Autodesk Inventor part; units mm, degrees
ref_plane "YZ Plane" through (0, 0, 0) normal (1, 0, 0) x (0, 1, 0)
ref_plane "XZ Plane" through (0, 0, 0) normal (0, 1, 0) x (-1, 0, 0)
ref_plane "XY Plane" through (0, 0, 0) normal (0, 0, 1) x (1, 0, 0)
sketch "Sketch1" plane through (0, 0, 0) normal (0, 1, 0) x (-1, 0, 0)
  line L0 (14.85, 7) -> (10.15, 7)
  line L1 (10.15, 7) -> (10.15, 2)
  line L2 (10.15, 2) -> (-10.15, 2)
  line L3 (-10.15, 2) -> (-10.15, 7)
  line L4 (-10.15, 7) -> (-14.85, 7)
  line L5 (-14.85, 7) -> (-14.85, 5)
  line L6 (-14.85, 5) -> (-12.15, 5)
  line L7 (-12.15, 5) -> (-12.15, 0)
  line L8 (-12.15, 0) -> (12.15, 0)
  line L9 (12.15, 0) -> (12.15, 5)
  line L10 (12.15, 5) -> (14.85, 5)
  line L11 (14.85, 5) -> (14.85, 7)
  point P0 (0, 0)
  point P1 (0, 0)
  point P2 (0, 2)
  point P3 (12.5, 7)
  point P4 (13.5, 5)
  dimension "d0" = 20.3
  dimension "d1" = 24.3
  dimension "d2" = 5
  dimension "d3" = 4.7
  dimension "d5" = 2
  dimension "d6" = 2
extrude "Extrusion1" add sketch "Sketch1" along normal mid plane 50
sketch "Sketch2" plane through (-10.15, 25, 2) normal (0, 0, 1) x (1, 0, 0)
  line L0 (13.1499, -10.0316) -> (13.1499, -19.0316)
  line L1 (7.1499, -19) -> (7.1499, -10)
  arc A0 (13.1499, -10.0316) -> (7.1499, -10) centre (10.15, -10) ccw
  arc A1 (7.1499, -19) -> (13.1499, -19.0316) centre (10.15, -19) ccw
  line L2 (0, 0) -> (20.3, 0)
  point P0 (10.15, -25)
  dimension "d9" = 6
  dimension "d12" = 9
  dimension "d13" = 10
extrude "Extrusion2" cut sketch "Sketch2" against normal up to surface (2 mm away)
pattern_linear "Rectangular Pattern1" count 2 spacing 25 along (0, -1, 0) of "Extrusion2"
properties part number "Part_B8"
Geometry check sheet. Reference: the model listing, model coordinates, mm. A direction names the side the tool comes from. Coordinates: 2 decimals unless noted, no trailing zeros. Write each loop counter-clockwise with the first axis right and the second up, starting at its lowest first coordinate (ties: lowest second). Pieces come first, ordered by that corner, then holes. Notation, with made-up numbers: M 87,-19 L 119,-19 A8 ccw 119,-9 Z; hole C 23.25,-4 d11. An arc over 180 degrees is marked long. One line per item, written item: value. Start each with the question number.
(1) Release check for a two-part mould opening along Y. For faces 5 (the face through (-1, -25, 1.7)), 6 (the face through (12.15, 0, 3)), 7 (the face through (0, -7, 1)) record: released by +Y, released by -Y, zero draft, split by the parting line, or undercut.
(2) Depth check by flat-ended pin: pin 1 (3 mm diameter, centred on x = 14, y = 8.5, fed in from -Z); pin 2 (1 mm diameter, centred on y = 12.5, z = 0.5, fed in from -X); pin 3 (4 mm diameter, centred on y = 8.5, z = 2.5, fed in from +X). Enter the tip coordinate at first touch or a pass-through.
(3) Tool access check on faces 1 (the face through (14, 0, 5)), 2 (the face through (-10.15, 0, 5)), 3 (the face through (0, 3, 1)), 4 (the face through (-12.15, 0, 2)). Record the directions out of +Z, -Z, +X, -X, +Y, -Y that give a thin tool (end or side, any length) a straight path to the whole face; none if there is none.
(4) Sectioned sample at A-A, the plane z = 1.25. Enter the section's corners in (x, y), and give its area (3 significant figures).
(5) Sectioned sample at D-D, the plane z = 6.25. Enter the section's corners in (x, y), and give its area (3 significant figures).
(6) Sectioned sample at B-B, the plane y = 7. Enter the section's corners in (x, z), and give its area (3 significant figures).
(7) Scan lines: line 1 along X through (y, z) = (-5, 4.25); line 2 along X through (y, z) = (16, 6.75); line 3 along Z through (x, y) = (-5, -14). Record each from-to range of solid material in increasing order. Write a range as [from, to].
(8) Sectioned sample at C-C, the plane x = 0. Enter the section's corners in (y, z).
Filled sheet:
1. face 5: released by -Y
1. face 6: zero draft
1. face 7: undercut
2. pin 1: z = 5
2. pin 2: x = -12.15
2. pin 3: x = 12.15
3. face 1: -Z, +X, +Y, -Y
3. face 2: +Z, +Y, -Y
3. face 3: +Z, -Z
3. face 4: -Z, -X, +Y, -Y
4. outline: M -12.15,-25 L 12.15,-25 L 12.15,25 L -12.15,25 Z; hole M -3,-19 A3 ccw 3,-19.03 L 3,-10.03 A3 ccw long -3,-10 Z; hole M -3,6 A3 ccw 3,5.97 L 3,14.97 A3 ccw long -3,15 Z
4. area: 1,050 mm²
5. outline: M -14.85,-25 L -10.15,-25 L -10.15,25 L -14.85,25 Z; M 10.15,-25 L 14.85,-25 L 14.85,25 L 10.15,25 Z
5. area: 470 mm²
6. outline: M -14.85,5 L -12.15,5 L -12.15,0 L -3,0 L -3,2 L -10.15,2 L -10.15,7 L -14.85,7 Z; M 3,0 L 12.15,0 L 12.15,5 L 14.85,5 L 14.85,7 L 10.15,7 L 10.15,2 L 3,2 Z
6. area: 67.4 mm²
7. line 1: [-12.15, -10.15], [10.15, 12.15]
7. line 2: [-14.85, -10.15], [10.15, 14.85]
7. line 3: [0, 2]
8. outline: M -25,0 L -22,0 L -22,2 L -25,2 Z; M -7,0 L 3,0 L 3,2 L -7,2 Z; M 18,0 L 25,0 L 25,2 L 18,2 Z
